```python
from build123d import *

# Parameters (mm, degrees)
F0_W     = 120
F0_H     = 60
F1_DEPTH = 44
F3_DEPTH = 16
F5_DEPTH = 15
F6_W     = 40
F6_H     = 12
F7_DEPTH = 60
F8_R     = 11
F9_DEPTH = 60.001


with BuildPart() as f1:
    # F0 (on Top) → F1 (new body)
    with BuildSketch(Plane.XY):
        with Locations((-26.462575, 17.752543)):
            Rectangle(F0_W, F0_H)
    extrude(amount=F1_DEPTH)

    # F2 (on face) → F3 (join)
    with BuildSketch(Plane.XY.offset(44)):
        with BuildLine():
            ThreePointArc((-61.462575, 3.752543), (-59.705216, -0.490098), (-55.462575, -2.247457))
            Line((-55.462575, -2.247457), (2.537425, -2.247457))
            ThreePointArc((2.537425, -2.247457), (6.780066, -0.490098), (8.537425, 3.752543))
            Line((8.537425, 3.752543), (8.537425, 31.752543))
            ThreePointArc((8.537425, 31.752543), (6.780066, 35.995184), (2.537425, 37.752543))
            Line((2.537425, 37.752543), (-55.462575, 37.752543))
            ThreePointArc((-55.462575, 37.752543), (-59.705216, 35.995184), (-61.462575, 31.752543))
            Line((-61.462575, 31.752543), (-61.462575, 3.752543))
        make_face()
    extrude(amount=F3_DEPTH)

    # F4 (on face) → F5 (cut)
    with BuildSketch(Plane.XY.offset(44)):
        with BuildLine():
            Line((33.537425, 2.752543), (33.537425, 32.752543))
            ThreePointArc((33.537425, 32.752543), (18.537425, 17.752543), (33.537425, 2.752543))
        make_face()
        with BuildLine():
            Line((-86.462575, 32.752543), (-86.462575, 2.752543))
            ThreePointArc((-86.462575, 2.752543), (-71.462575, 17.752543), (-86.462575, 32.752543))
        make_face()
    extrude(amount=-F5_DEPTH, mode=Mode.SUBTRACT)

    # F6 (on face) → F7 (cut)
    with BuildSketch(Plane.XZ.offset(12.247457)):
        with Locations((-26.462575, 6)):
            Rectangle(F6_W, F6_H)
    extrude(amount=-F7_DEPTH, mode=Mode.SUBTRACT)

    # F8 (on face) → F9 (cut, through all)
    with BuildSketch(Plane.XY.offset(60)):
        with Locations((-26.462575, 17.752543)):
            Circle(F8_R)
    extrude(amount=-F9_DEPTH, mode=Mode.SUBTRACT)


solid = f1.part
```
Design review of the part built by this model. Coordinates are the model's own, in mm. A direction names the side the tool comes from. Give positions to 0.01 mm unless a question says otherwise; leave off trailing zeros. Order: outer loops, then holes, each group sorted by start corner. A loop starts at its lowest first (then second) coordinate and runs counter-clockwise, first axis right, second up. Notation, with made-up numbers: (4.5, 40) -> (40.5, 40) arc R29 ccw to (40.5, 65) -> close; hole circle Ø3 at (-34.5, 66). An arc over 180 degrees is marked (long way). Write each question's results on one line, items separated by ' | '. Start each with the question number.
Q1. Machinability: for faces 1 (the cylindrical face through (6.73, -0.54, 51.89)), 2 (the cylindrical face through (-59.7, 36, 51.9)), 3 (the cylindrical face through (-59.752, -0.443, 51.888)), 4 (the flat face through (-61.463, 18, 52)), 5 (the cylindrical face through (-71.466, 17.423, 36.605)), which of the approach directions +Z, -Z, +X, -X, +Y, -Y give a long, thin tool a straight path to every point of the face, cutting with its end or side? Answer none if there is none.
Q2. Add section C-C on y = 39.5. Give the boundary of the cut face in (x, z), and give its area (3 significant figures).
Q3. Add section A-A on x = -51. Give the boundary of the cut face in (y, z), and give its area (3 significant figures).
Q4. Wall thickness on L1, parallel to X at y = -1.5, z = 7; L2, parallel to Y at x = -11.5, z = 55; L3, parallel to X at y = 16, z = 34: over which ranges is each line inside the solid? List them lowest first. Write a range as from..to.
Q5. Add section D-D on x = -25. Give the boundary of the cut face in (y, z).
Q6. For pin 1 (5 mm diameter, centred on y = 14, z = 49, fed in from -X); pin 2 (16.5 mm diameter, centred on x = 23, y = 10.5, fed in from +Z); pin 3 (12 mm diameter, centred on x = -32, y = 9, fed in from -Z), all flat-tipped, find the tip position at first contact; note any pin that passes through.
Q7. Add section B-B on z = 10.5. Give the boundary of the cut face in (x, y), and give its area (3 significant figures).
Q8. Mouldability with a two-part tool opening along Y and no side actions: class faces 6 (the flat face through (-26, 37.753, 52)), 7 (the flat face through (-81, 18, 29)), 8 (the flat face through (-6.463, 17, 6)) as +Y half, -Y half, draft (parallel to the pull), parting line (faces both ways), or undercut.
Found:
1) face 1: +Z, +X, -Y | face 2: +Z, -X, +Y | face 3: +Z, -X, -Y | face 4: +Z, -X, +Y, -Y | face 5: +Z, -X
2) outline: (-86.46, 0) -> (-46.46, 0) -> (-46.46, 12) -> (-6.46, 12) -> (-6.46, 0) -> (33.54, 0) -> (33.54, 44) -> (-86.46, 44) -> close | area: 4,800 mm2
3) outline: (-12.25, 0) -> (47.75, 0) -> (47.75, 44) -> (37.75, 44) -> (37.75, 60) -> (-2.25, 60) -> (-2.25, 44) -> (-12.25, 44) -> close | area: 3,280 mm2
4) L1: x = -86.46..-46.46, -6.46..33.54 | L2: y = -2.25..37.75 | L3: x = -71.57..-37.32, -15.6..18.64
5) outline: (-12.25, 12) -> (6.85, 12) -> (6.85, 60) -> (-2.25, 60) -> (-2.25, 44) -> (-12.25, 44) -> close; (28.65, 12) -> (47.75, 12) -> (47.75, 44) -> (37.75, 44) -> (37.75, 60) -> (28.65, 60) -> close
6) pin 1: stops at x = -61.46 | pin 2: stops at z = 44 | pin 3: stops at z = 12
7) outline: (-86.46, -12.25) -> (-46.46, -12.25) -> (-46.46, 47.75) -> (-86.46, 47.75) -> close; (-6.46, -12.25) -> (33.54, -12.25) -> (33.54, 47.75) -> (-6.46, 47.75) -> close | area: 4,800 mm2
8) face 6: +Y half | face 7: undercut | face 8: draft
